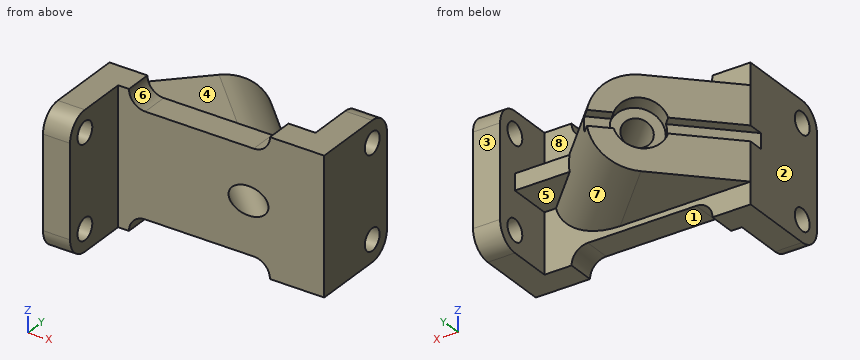
```python
from build123d import *

# Parameters (mm, degrees)
BOSS_EXTRUDE1_DEPTH = 62.5
FILLET1_R           = 20
SKETCH2_R           = 10
CUT_EXTRUDE1_DEPTH  = 240.491649124
SKETCH3_R           = 10
CUT_EXTRUDE2_DEPTH  = 125
SKETCH4_W           = 148.086919985
SKETCH4_H           = 40
BOSS_EXTRUDE2_DEPTH = 7.5
BOSS_EXTRUDE3_REACH = 243.312
CUT_EXTRUDE3_REACH  = 221.395
CUT_EXTRUDE4_DEPTH  = 10


with BuildPart() as part:
    # Sketch1 → Boss-Extrude1 (new, symmetric)
    with BuildSketch(Plane.XY):
        Polygon((0, 0), (190, 0), (190, 85), (165, 85), (165, 25), (-25, 25), (-25, -65), (0, -65), align=None)
    extrude(amount=BOSS_EXTRUDE1_DEPTH, both=True)

    # Fillet1
    fillet1_edges = [part.edges().sort_by_distance(p)[0] for p in [
        (177.5, 85, -62.5),
        (177.5, 85, 62.5),
        (-12.5, -65, 62.5),
        (-12.5, -65, -62.5),
    ]]
    fillet(fillet1_edges, radius=FILLET1_R)

    # Sketch2 → Cut-Extrude1 (cut, through all)
    with BuildSketch(Plane(origin=(190, 0, 0), x_dir=(0, 0, -1), z_dir=(1, 0, 0))):
        with Locations((42.5, 65)):
            Circle(SKETCH2_R)
        with Locations((-42.5, 65)):
            Circle(SKETCH2_R)
    extrude(amount=-CUT_EXTRUDE1_DEPTH, mode=Mode.SUBTRACT)

    # Sketch3 → Cut-Extrude2 (cut)
    with BuildSketch(Plane.ZY.offset(25)):
        with Locations(Location((42.5, -45, 0), (0, 0, 270))):
            Circle(SKETCH3_R)
        with Locations(Location((-42.5, -45, 0), (0, 0, 270))):
            Circle(SKETCH3_R)
    extrude(amount=-CUT_EXTRUDE2_DEPTH, mode=Mode.SUBTRACT)

    # Sketch4 → Boss-Extrude2 (add, symmetric)
    with BuildSketch(Plane.XY):
        with Locations((90.956540007, 45)):
            Rectangle(SKETCH4_W, SKETCH4_H)
    extrude(amount=BOSS_EXTRUDE2_DEPTH, both=True)

    # Sketch5 → Boss-Extrude3 (add, up to next)
    with BuildSketch(Plane(origin=(-25, 25, 0), x_dir=(0, 0, -1), z_dir=(-0.707106781186549, 0.7071067811865461, 0)), mode=Mode.PRIVATE) as boss_extrude3_sk1:
        with BuildLine():
            Line((-42.5, 0), (-42.5, -85))
            ThreePointArc((-42.5, -85), (0, -127.5), (42.5, -85))
            Line((42.5, -85), (42.5, 0))
            Line((42.5, 0), (-42.5, 0))
        make_face()
    boss_extrude3_tool1 = extrude(boss_extrude3_sk1.sketch, amount=-BOSS_EXTRUDE3_REACH, mode=Mode.PRIVATE) - part.part
    add(boss_extrude3_tool1.solids().sort_by_distance((17.122184, 67.122184, 0))[0])

    # Sketch7 → Cut-Extrude3 (cut, up to next)
    with BuildSketch(Plane(origin=(0, 25, 0), x_dir=(1, 0, 0), z_dir=(0, 1, 0)), mode=Mode.PRIVATE) as cut_extrude3_sk1:
        with BuildLine():
            Line((25, -47.5), (125, -47.5))
            ThreePointArc((125, -47.5), (135.606601718, -51.893398282), (140, -62.5))
            Line((140, -62.5), (10, -62.5))
            ThreePointArc((10, -62.5), (14.393398282, -51.893398282), (25, -47.5))
        make_face()
    cut_extrude3_tool1 = extrude(cut_extrude3_sk1.sketch, amount=-CUT_EXTRUDE3_REACH, mode=Mode.PRIVATE) & part.part
    cut_extrude3 = cut_extrude3_tool1.solids().sort_by_distance((75, 25, 55.216204))[0]
    add(cut_extrude3, mode=Mode.SUBTRACT)

    # Mirror1: Cut-Extrude3 across plane
    add(cut_extrude3.mirror(Plane.XY), mode=Mode.SUBTRACT)

    # Sketch8 → Cut-Extrude4 (cut)
    with BuildSketch(Plane(origin=(-25, 25, 0), x_dir=(0, 0, 1), z_dir=(-0.7071067811865489, 0.7071067811865462, 0))):
        with BuildLine():
            Line((-7, -26.74015117), (-7, 126.919565837))
            ThreePointArc((-7, 126.919565837), (0, 127.5), (7, 126.919565837))
            Line((7, 126.919565837), (7, -26.74015117))
            Line((7, -26.74015117), (-7, -26.74015117))
        make_face()
    extrude(amount=-CUT_EXTRUDE4_DEPTH, mode=Mode.SUBTRACT)

    # Sketch13 → CBORE for M24 Hex Head Bolt2 (revolve, cut)
    with BuildSketch(Plane(origin=(35.104076401, 85.104076401, 0), x_dir=(-0.7071067811865462, -0.7071067811865489, 0), z_dir=(0, 0, 1))):
        Polygon((0, 0), (0, 215.667568262), (13, 215.667568262), (13, 15.9), (22.285, 15.9), (22.285, 0.025), (22.31, 0), align=None)
    revolve(axis=Axis((30.61394834, 89.594204461, 0), (0.7071067811865489, -0.7071067811865462, 0)), mode=Mode.SUBTRACT)


solid = part.part
```
Geometry check sheet. Reference: the model listing, model coordinates, mm. Face numbers are marked on the shaded views. A direction names the side the tool comes from. Coordinates: 2 decimals unless noted, no trailing zeros. Order: outer loops, then holes, each group sorted by start corner. A loop starts at its lowest first (then second) coordinate and runs counter-clockwise, first axis right, second up. Notation, with made-up numbers: (17, 77) - (43, 77) arc R30 ccw to (43, 113) - close; hole circle Ø3 at (-19, 80.25). An arc over 180 degrees is marked (long way). Use one line per item in the form item = value.
1. Access from +Z, -Z, +X, -X, +Y, -Y to the whole of each face (thin tool, end or side, straight path). Record for the marked faces 4, 5, 6, 7 and 8.
Here are the results:
face_4 = +Z, -X, +Y
face_5 = -Z, +Y
face_6 = +Z, +Y, -Y
face_7 = +Y
face_8 = +Z, +Y
2. Scan lines: line 1 (Z direction, x = -10.25, y = -45); line 2 (X direction, y = 59, z = 11); line 3 (Y direction, x = 175, z = -42). Record each from-to range of solid material in increasing order.
Here are the results:
line_1 = -62.5 to -52.5, -32.5 to 32.5, 52.5 to 62.5
line_2 = 9 to 51.41, 71.01 to 119.26, 165 to 190
line_3 = 0 to 55.01, 74.99 to 85
3. Section check B-B (z = 26). Record the boundary of the cut face in (x, y), then the cut area to 3 significant figures.
Here are the results:
outline = (-25, -65) - (0, -65) - (0, 0) - (190, 0) - (190, 85) - (165, 85) - (165, 25) - (142.75, 25) - (58.88, 108.88) - (-25, 25) - close
area = 15,500 mm²
4. Gauge pin test, flat ends, axial feed: pin 1 (10 mm diameter, centred on x = 44, y = 51, fed in from +Z); pin 2 (8 mm diameter, centred on y = 65.5, z = -33.5, fed in from -X); pin 3 (5 mm diameter, centred on x = 103.5, y = 30.5, fed in from +Z). Record the tip position at first contact, or that the pin passes through.
Here are the results:
pin_1 = 42.5
pin_2 = 11.5
pin_3 = 41.88
5. Section check C-C (y = -13). Record the boundary of the cut face in (x, z), then the cut area to 4 significant figures.
Here are the results:
outline = (-25, -62.5) - (0, -62.5) - (0, 62.5) - (-25, 62.5) - close
area = 3,125 mm²
6. Draft check along X on the marked faces 1, 2 and 3. Enter one of: pulls with the +X half, pulls with the -X half, needs draft (parallel to the pull), parting line crosses it, or undercut.
Here are the results:
face_1 = undercut
face_2 = pulls with the -X half
face_3 = needs draft
7. Section check A-A (y = -48). Record the boundary of the cut face in (x, z), then the cut area to 3 significant figures.
Here are the results:
outline = (-25, -62.27) - (0, -62.27) - (0, -52.04) - (-25, -52.04) - close; (-25, -32.96) - (0, -32.96) - (0, 32.96) - (-25, 32.96) - close; (-25, 52.04) - (0, 52.04) - (0, 62.27) - (-25, 62.27) - close
area = 2,160 mm²
